from build123d import *

# Parameters (mm, degrees)
EXTRUDE_1_DEPTH     = 50
SKETCH_2_R          = 1.5
EXTRUDE_2_DEPTH     = 4
SKETCH_3_R          = 1.5
CUT_EXTRUDE_1_DEPTH = 4
CHAMFER_1_SIZE      = 0.2
FILLET_1_R          = 0.1


with BuildPart() as part:
    # 草图1 → 凸台-拉伸1 (new body)
    with BuildSketch(Plane(origin=(0, 0, 0), x_dir=(1, 0, 0), z_dir=(0, 1, 0))):
        Polygon((2.713546265, 0), (1.356773133, 2.35), (-1.356773133, 2.35), (-2.713546265, 0), (-1.356773133, -2.35), (1.356773133, -2.35), align=None)
    extrude(amount=EXTRUDE_1_DEPTH)

    # 草图2 → 凸台-拉伸2 (add)
    with BuildSketch(Plane(origin=(0, 50, 0), x_dir=(1, 0, 0), z_dir=(0, 1, 0))):
        Circle(SKETCH_2_R)
    extrude(amount=EXTRUDE_2_DEPTH)

    # 草图3 → 切除-拉伸1 (cut)
    with BuildSketch(Plane.XZ):
        Circle(SKETCH_3_R)
    extrude(amount=-CUT_EXTRUDE_1_DEPTH, mode=Mode.SUBTRACT)

    # 倒角1
    chamfer_1_edges = [part.edges().sort_by_distance(p)[0] for p in [
        (-1.5, 4, 0),
        (-1.5, 54, 0),
    ]]
    chamfer(chamfer_1_edges, length=CHAMFER_1_SIZE)

    # 圆角1
    fillet_1_edges = [part.edges().sort_by_distance(p)[0] for p in [
        (2.713546265, 25, 0),
        (1.356773133, 25, -2.35),
        (1.356773133, 25, 2.35),
        (-1.356773133, 25, -2.35),
        (-1.356773133, 25, 2.35),
        (-2.713546265, 25, 0),
    ]]
    fillet(fillet_1_edges, radius=FILLET_1_R)


solid = part.part
Read the model definition and answer for the solid it produces. Units are mm, in the model's axes. A direction names the side the tool comes from. Coordinates: 2 decimals unless noted, no trailing zeros. Order: outer loops, then holes, each group sorted by start corner. A loop starts at its lowest first (then second) coordinate and runs counter-clockwise, first axis right, second up. Notation, with made-up numbers: (-21, 57.25) -> (-16, 57.25) arc R14 ccw to (-16, 77.25) -> close; hole circle Ø2 at (20.25, -25.5). An arc over 180 degrees is marked (long way). Answer as a JSON object with one key per item and string values.
1) A cutting plane is placed at B-B, the plane y = 13. Determine the outline of the cut face in (x, z), plus the area to 3 significant figures.
Model answer:
{"outline": "(-2.68, -0.05) -> (-1.39, -2.3) arc R0.1 ccw to (-1.3, -2.35) -> (1.3, -2.35) arc R0.1 ccw to (1.39, -2.3) -> (2.68, -0.05) arc R0.1 ccw to (2.68, 0.05) -> (1.39, 2.3) arc R0.1 ccw to (1.3, 2.35) -> (-1.3, 2.35) arc R0.1 ccw to (-1.39, 2.3) -> (-2.68, 0.05) arc R0.1 ccw to start", "area": "19.1 mm²"}
2) Consider line 1 along Z through (x, y) = (0, 1.8); line 2 along Y through (x, z) = (0.5, -1.85); line 3 along Y through (x, z) = (0.8, 0.85). Determine where each line is inside the solid, lowest interval first. Write a range as from..to.
Model answer:
{"line 1": "z = -2.35..-1.5, 1.5..2.35", "line 2": "y = 0..50", "line 3": "y = 4..54"}
3) The mould has two halves that part along Z. Classify faces 3 (the face through (-2.044, 24.65, 1.159)), 4 (the face through (-1.5, 1.87, 0.07)), 5 (the face through (0, 4, 0)), 6 (the face through (0, 0, -2)): released by +Z, released by -Z, zero draft, split by the parting line, or undercut.
Model answer:
{"face 3": "released by +Z", "face 4": "undercut", "face 5": "undercut", "face 6": "zero draft"}
4) A tool of negligible diameter and unlimited length cuts with its end or side. For faces 1 (the face through (-1.5, 51.87, -0.07)), 2 (the face through (-2.026, 24.65, -1.191)), from which of +Z, -Z, +X, -X, +Y, -Y can it reach the whole face along a straight path? Write none if from no direction.
Model answer:
{"face 1": "+Y", "face 2": "-Z, -X, +Y, -Y"}
5) Each of these flat-tipped pins is pushed along its axis until it touches: pin 1 (1.5 mm diameter, centred on y = 40.5, z = 1.5, fed in from +X); pin 2 (1 mm diameter, centred on x = 1.5, z = 1.5, fed in from +Y); pin 3 (1 mm diameter, centred on x = 2, y = 43.5, fed in from -Z). Where does it stop, or does it pass through?
Model answer:
{"pin 1": "stops at x = 2.28", "pin 2": "stops at y = 50", "pin 3": "stops at z = -2.1"}
6) A cutting plane is placed at A-A, the plane x = 0. Determine the outline of the cut face in (y, z), plus the area to 3 significant figures.
Model answer:
{"outline": "(0, -2.35) -> (50, -2.35) -> (50, -1.5) -> (53.8, -1.5) -> (54, -1.3) -> (54, 1.3) -> (53.8, 1.5) -> (50, 1.5) -> (50, 2.35) -> (0, 2.35) -> (0, 1.5) -> (3.8, 1.5) -> (4, 1.3) -> (4, -1.3) -> (3.8, -1.5) -> (0, -1.5) -> close", "area": "235 mm²"}
7) A cutting plane is placed at C-C, the plane x = 2.2. Determine the outline of the cut face in (y, z).
Model answer:
{"outline": "(0, -0.89) -> (50, -0.89) -> (50, 0.89) -> (0, 0.89) -> close"}
